from build123d import *

# Parameters (mm, degrees)
ESQUISSE1_R             = 7
BOSS_EXTRU_1_DEPTH      = 44
ESQUISSE1_4_R           = 7
ENL_V_MAT_EXTRU_1_DEPTH = 19
ENL_V_START             = -8
ESQUISSE1_5_R           = 5.5
ENL_V_MAT_EXTRU_2_DEPTH = 24
ESQUISSE1_7_R           = 5.5
ENL_V_MAT_EXTRU_3_DEPTH = 45
ENL_V_MAT_EXTRU_4_DEPTH = 32
ESQUISSE1_12_R          = 5.5
ENL_V_MAT_EXTRU_5_DEPTH = 7


with BuildPart() as part:
    # Esquisse1 → Boss.-Extru.1 (new body)
    with BuildSketch(Plane.XY):
        with BuildLine():
            Line((0, 0), (29, 34))
            Line((29, 34), (29, 53))
            Line((29, 53), (24, 58))
            Line((24, 58), (0, 58))
            ThreePointArc((0, 58), (-8.438901294, 48.982044142), (-20.638619164, 47.057085233))
            Line((-20.638619164, 47.057085233), (-43, 51))
            Line((-43, 51), (-50, 51))
            Line((-50, 51), (-57, 44))
            Line((-57, 44), (-57, 26))
            Line((-57, 26), (-50, 19))
            Line((-50, 19), (-17.424461089, 19))
            ThreePointArc((-17.424461089, 19), (-14.159225308, 17.786586232), (-12.478822347, 14.735294118))
            ThreePointArc((-12.478822347, 14.735294118), (-10.141992144, 6.884327939), (-5.703019947, 0))
            Line((-5.703019947, 0), (0, 0))
        make_face()
        with Locations((-43, 33)):
            Circle(ESQUISSE1_R, mode=Mode.SUBTRACT)
    extrude(amount=-BOSS_EXTRU_1_DEPTH)

    # Esquisse1_4 → Enl_v. mat.-Extru.1 (cut)
    with BuildSketch(Plane.XY):
        with BuildLine():
            Line((-5.703019947, 0), (0, 0))
            Line((0, 0), (16.205882353, 19))
            Line((16.205882353, 19), (-17.424461089, 19))
            ThreePointArc((-17.424461089, 19), (-14.159225308, 17.786586232), (-12.478822347, 14.735294118))
            ThreePointArc((-12.478822347, 14.735294118), (-10.141992144, 6.884327939), (-5.703019947, 0))
        make_face()
        Polygon((-50, 19), (-23, 19), (-23, 47.473460386), (-43, 51), (-50, 51), (-57, 44), (-57, 26), align=None)
        with Locations((-43, 33)):
            Circle(ESQUISSE1_4_R, mode=Mode.SUBTRACT)
    extrude(amount=-ENL_V_MAT_EXTRU_1_DEPTH, mode=Mode.SUBTRACT)

    # Esquisse1_5 → Enl_v. mat.-Extru.2 (cut)
    with BuildSketch(Plane.XY.offset(ENL_V_START)):
        with BuildLine():
            ThreePointArc((-9.425038644, 47.400950208), (1.146296181, 31.615810491), (17.698037548, 22.290382158))
            Line((17.698037548, 22.290382158), (28, 34.368545033))
            Line((28, 34.368545033), (28, 52.585786438))
            Line((28, 52.585786438), (23.585786438, 57))
            Line((23.585786438, 57), (0.636084685, 57))
            ThreePointArc((0.636084685, 57), (-3.53336375, 51.297910101), (-9.425038644, 47.400950208))
        make_face()
        with Locations((15, 44)):
            Circle(ESQUISSE1_5_R, mode=Mode.SUBTRACT)
        with BuildLine():
            ThreePointArc((17.698037548, 22.290382158), (18.23039297, 22.141595828), (18.764705882, 22))
            Line((18.764705882, 22), (29, 34))
            Line((29, 34), (29, 53))
            Line((29, 53), (24, 58))
            Line((24, 58), (0, 58))
            ThreePointArc((0, 58), (-3.978755657, 52.259333621), (-9.763063451, 48.344294617))
            ThreePointArc((-9.763063451, 48.344294617), (-9.59693318, 47.871589669), (-9.425038644, 47.400950208))
            ThreePointArc((-9.425038644, 47.400950208), (-3.53336375, 51.297910101), (0.636084685, 57))
            Line((0.636084685, 57), (23.585786438, 57))
            Line((23.585786438, 57), (28, 52.585786438))
            Line((28, 52.585786438), (28, 34.368545033))
            Line((28, 34.368545033), (17.698037548, 22.290382158))
        make_face()
    extrude(amount=-ENL_V_MAT_EXTRU_2_DEPTH, mode=Mode.SUBTRACT)

    # Esquisse1_7 → Enl_v. mat.-Extru.3 (cut, through all)
    with BuildSketch(Plane.XY):
        with Locations((15, 44)):
            Circle(ESQUISSE1_7_R)
    extrude(amount=-ENL_V_MAT_EXTRU_3_DEPTH, mode=Mode.SUBTRACT)

    # Esquisse1_11 → Enl_v. mat.-Extru.4 (cut)
    with BuildSketch(Plane.XY):
        with BuildLine():
            Line((15.744476296, 20), (16.986847747, 21.456573425))
            ThreePointArc((16.986847747, 21.456573425), (0.310181683, 31.027872638), (-10.353317057, 47.028208705))
            ThreePointArc((-10.353317057, 47.028208705), (-15.518923584, 45.851449437), (-20.812267342, 46.07227748))
            Line((-20.812267342, 46.07227748), (-22, 46.281706793))
            Line((-22, 46.281706793), (-22, 20))
            Line((-22, 20), (-17.424461089, 20))
            Line((-17.424461089, 20), (15.744476296, 20))
        make_face()
    extrude(amount=-ENL_V_MAT_EXTRU_4_DEPTH, mode=Mode.SUBTRACT)

    # Esquisse1_12 → Enl_v. mat.-Extru.5 (cut)
    with BuildSketch(Plane.XY):
        with BuildLine():
            ThreePointArc((-9.425038644, 47.400950208), (1.146296181, 31.615810491), (17.698037548, 22.290382158))
            Line((17.698037548, 22.290382158), (28, 34.368545033))
            Line((28, 34.368545033), (28, 52.585786438))
            Line((28, 52.585786438), (23.585786438, 57))
            Line((23.585786438, 57), (0.636084685, 57))
            ThreePointArc((0.636084685, 57), (-3.53336375, 51.297910101), (-9.425038644, 47.400950208))
        make_face()
        with Locations((15, 44)):
            Circle(ESQUISSE1_12_R, mode=Mode.SUBTRACT)
        with BuildLine():
            Line((16.986847747, 21.456573425), (17.698037548, 22.290382158))
            ThreePointArc((17.698037548, 22.290382158), (1.146296181, 31.615810491), (-9.425038644, 47.400950208))
            ThreePointArc((-9.425038644, 47.400950208), (-9.88684711, 47.208774961), (-10.353317057, 47.028208705))
            ThreePointArc((-10.353317057, 47.028208705), (0.310181683, 31.027872638), (16.986847747, 21.456573425))
        make_face()
    extrude(amount=-ENL_V_MAT_EXTRU_5_DEPTH, mode=Mode.SUBTRACT)


solid = part.part
Read the model definition and answer for the solid it produces. Units are mm, in the model's axes. A direction names the side the tool comes from. Give positions to 0.01 mm unless a question says otherwise; leave off trailing zeros. Write each loop counter-clockwise with the first axis right and the second up, starting at its lowest first coordinate (ties: lowest second). Pieces come first, ordered by that corner, then holes. Notation, with made-up numbers: (23, 40) - (56, 40) arc R24 cw to (56, 55) - close; hole circle Ø3 at (13.5, 83.25). An arc over 180 degrees is marked (long way). Return JSON: item names as keys, results as strings.
Q1. Consider line 1 along Z through (x, y) = (24, 41); line 2 along Y through (x, z) = (-43, -34); line 3 along X through (y, z) = (31.5, -20). Determine where each line is inside the solid, lowest interval first. Write a range as [from, to].
Reply:
{"line 1": "[-44, -32], [-8, -7]", "line 2": "[19, 26], [40, 51]", "line 3": "[-57, -49.84], [-36.16, -22], [-0.19, 1.27]"}
Q2. A cutting plane is placed at C-C, the plane x = -40. Determine the outline of the cut face in (y, z), and give its area (3 significant figures).
Reply:
{"outline": "(19, -44) - (26.68, -44) - (26.68, -19) - (19, -19) - close; (39.32, -44) - (50.47, -44) - (50.47, -19) - (39.32, -19) - close", "area": "471 mm²"}
Q3. A cutting plane is placed at B-B, the plane y = 27. Determine the outline of the cut face in (x, z), and give its area (3 significant figures).
Reply:
{"outline": "(-57, -44) - (-46.61, -44) - (-46.61, -19) - (-57, -19) - close; (-39.39, -44) - (23.03, -44) - (23.03, -32) - (7.16, -32) - (7.16, -8) - (23.03, -8) - (23.03, 0) - (21.72, 0) - (21.72, -7) - (5.34, -7) - (5.34, -32) - (-22, -32) - (-22, 0) - (-23, 0) - (-23, -19) - (-39.39, -19) - close", "area": "1,320 mm²"}
Q4. Given P1, Ø9.5, axis at x = -6, y = 8.5, coming from the +Z side; P2, Ø6, axis at x = -35, z = -35.5, coming from the -Y side; P3, Ø12.5, axis at x = 15, y = 44, coming from the +Z side; P4, Ø11, axis at x = 17, y = 44.5, coming from the -Z side, each flat-ended and moving along its own axis, determine where each tip first touches the part or whether it passes through.
Reply:
{"P1": "z = -19", "P2": "y = 19", "P3": "z = -7", "P4": "z = -44"}
Q5. For faces 4 (the face through (-36, 39, -19)), 5 (the face through (-31.66, 49, -31.47)), 6 (the face through (-46, 51, -31)), 7 (the face through (-11, 31, -32)), determine the directions among +Z, -Z, +X, -X, +Y, -Y from which every point of the face is accessible in a straight line to the end or side of a thin tool.
Reply:
{"face 4": "+Z, -X, +Y, -Y", "face 5": "+Z, -Z, +Y", "face 6": "+Z, -Z, -X, +Y", "face 7": "+Z"}
Q6. A cutting plane is placed at D-D, the plane y = 33. Determine the outline of the cut face in (x, z).
Reply:
{"outline": "(-57, -44) - (-50, -44) - (-50, -19) - (-57, -19) - close; (-36, -44) - (28.15, -44) - (28.15, -32) - (-0.28, -32) - (-0.28, -8) - (28.15, -8) - (28.15, 0) - (26.83, 0) - (26.83, -7) - (-1.66, -7) - (-1.66, -32) - (-22, -32) - (-22, 0) - (-23, 0) - (-23, -19) - (-36, -19) - close"}
Q7. For a pull along X with two mould halves and no side action, classify faces 1 (the face through (12, 58, -4)), 2 (the face through (12, 57, -3)), 3 (the face through (-53, 48, -31)) as released by +X, released by -X, zero draft, split by the parting line, or undercut.
Reply:
{"face 1": "zero draft", "face 2": "undercut", "face 3": "released by -X"}
Q8. A cutting plane is placed at A-A, the plane z = -23.5. Determine the outline of the cut face in (x, y).
Reply:
{"outline": "(-57, 26) - (-50, 19) - (-17.42, 19) arc R5 cw to (-12.48, 14.74) arc R29 ccw to (-5.7, 0) - (0, 0) - (18.76, 22) arc R41 cw to (17.7, 22.29) arc R41 cw to (-9.43, 47.4) arc R41 cw to (-9.76, 48.34) arc R19 cw to (-20.64, 47.06) - (-43, 51) - (-50, 51) - (-57, 44) - close; hole circle Ø14 at (-43, 33); hole (-22, 20) - (15.74, 20) - (16.99, 21.46) arc R42 cw to (-10.35, 47.03) arc R20 cw to (-20.81, 46.07) - (-22, 46.28) - close"}
